```python
from build123d import *

# Parameters (mm, degrees)
SKETCH1_R           = 7.4
BOSS_EXTRUDE1_DEPTH = 3.5
SKETCH2_R           = 4
BOSS_EXTRUDE2_DEPTH = 2.25
FILLET1_R           = 1.5
FILLET2_R           = 1.5


with BuildPart() as part:
    # Sketch1 → Boss-Extrude1 (new body)
    with BuildSketch(Plane.XY):
        with Locations((-48.895186784, 18.701845636)):
            Circle(SKETCH1_R)
    extrude(amount=BOSS_EXTRUDE1_DEPTH)

    # Sketch2 → Boss-Extrude2 (add)
    with BuildSketch(Plane(origin=(0, 0, 0), x_dir=(-1, 0, 0), z_dir=(0, 0, -1))):
        with Locations((48.895186784, 18.701845636)):
            Circle(SKETCH2_R)
    extrude(amount=BOSS_EXTRUDE2_DEPTH)

    # Fillet1
    fillet1_edges = [part.edges().sort_by_distance(p)[0] for p in [
        (-56.295186784, 18.701845636, 3.5),
    ]]
    fillet(fillet1_edges, radius=FILLET1_R)

    # Fillet2
    fillet2_edges = [part.edges().sort_by_distance(p)[0] for p in [
        (-56.295186784, 18.701845636, 0),
    ]]
    fillet(fillet2_edges, radius=FILLET2_R)


solid = part.part
```
CAD build for the part. Positions are in the model's coordinates, mm. Round coordinates to 2 decimals unless told otherwise and drop trailing zeros. Order: outer loops, then holes, each group sorted by start corner. A loop starts at its lowest first (then second) coordinate and runs counter-clockwise, first axis right, second up. Notation, with made-up numbers: (24.5, 66) - (29.5, 66) arc R13 cw to (29.5, 87) - close; hole circle Ø7 at (52, 42.5). An arc over 180 degrees is marked (long way). Answer in a Markdown table with one row per item. Add a question column.
(1) Band-saw the part on A-A on z = 2.4. List the corners of the cut face in (x, y).
(2) Mould opens along Z. For faces 1 (the face through (-56.288, 19.027, 1.746)), 2 (the face through (-49, 19, 3.5)), 3 (the face through (-49, 19, -2.25)) say: +Z half, -Z half, draft (parallel to the pull), parting line (faces both ways), or undercut.
(3) Band-saw the part on B-B on z = -1.5. List the corners of the cut face in (x, y), and give its area (3 significant figures).
(4) Drop a flat-ended pin along its axis: pin 1 Ø3 at (y, z) = (20.5, 1.5) entering from +X. Give the stop position or say it passes through.
(5) Probe L1, parallel to Z at x = -44.25, y = 20.5; L2, parallel to Y at x = -47.5, z = 1.6; L3, parallel to X at y = 24.5, z = 2.7. List the from-to ranges inside material, lowest first. Write a range as [from, to].
Data:
| question | item | result |
|---|---|---|
| 1 | outline | circle Ø14.69 at (-48.9, 18.7) |
| 2 | face 1 | draft |
| 2 | face 2 | +Z half |
| 2 | face 3 | -Z half |
| 3 | outline | circle Ø8 at (-48.9, 18.7) |
| 3 | area | 50.3 mm^2 |
| 4 | pin 1 | stops at x = -41.5 |
| 5 | L1 | z = [0, 3.5] |
| 5 | L2 | y = [11.43, 25.97] |
| 5 | L3 | x = [-53.21, -44.58] |
